```python
from build123d import *

# Parameters (mm, degrees)
CROQUIS1_R              = 8
SALIENTE_EXTRUIR1_DEPTH = 80
CROQUIS2_R              = 11
SALIENTE_EXTRUIR2_DEPTH = 20
CHAFL_N1_SIZE           = 2
CHAFL_N2_SIZE           = 2


with BuildPart() as part:
    # Croquis1 → Saliente-Extruir1 (new body)
    with BuildSketch(Plane(origin=(0, 0, 0), x_dir=(1, 0, 0), z_dir=(0, 1, 0))):
        Circle(CROQUIS1_R)
    extrude(amount=SALIENTE_EXTRUIR1_DEPTH)

    # Croquis2 → Saliente-Extruir2 (add, symmetric)
    with BuildSketch(Plane(origin=(0, 40, 0), x_dir=(1, 0, 0), z_dir=(0, 1, 0))):
        Circle(CROQUIS2_R)
    extrude(amount=SALIENTE_EXTRUIR2_DEPTH, both=True)

    # Chaflán1
    chafl_n1_edges = [part.edges().sort_by_distance(p)[0] for p in [
        (-8, 80, 0),
    ]]
    chamfer(chafl_n1_edges, length=CHAFL_N1_SIZE)

    # Chaflán2
    chafl_n2_edges = [part.edges().sort_by_distance(p)[0] for p in [
        (-8, 0, 0),
    ]]
    chamfer(chafl_n2_edges, length=CHAFL_N2_SIZE)


solid = part.part
```
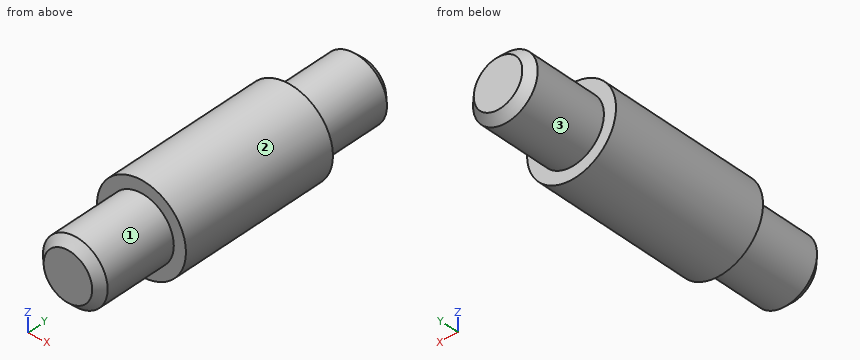
The model under review builds one solid part; all positions refer to its coordinate system, in mm. Face numbers are marked on the shaded views. A direction names the side the tool comes from. Round coordinates to 2 decimals unless told otherwise and drop trailing zeros. Write each loop counter-clockwise with the first axis right and the second up, starting at its lowest first coordinate (ties: lowest second). Pieces come first, ordered by that corner, then holes. Notation, with made-up numbers: M 52.5,-8 L 107.5,-8 A7 cw 107.5,5 Z; hole C 78,79 d8. An arc over 180 degrees is marked long. Use CSV: the item, a comma, the result in double quotes. Start each with the question number.
(1) We need section D-D, the plane y = 23. State the section outline as (x, z) points.
(2) We need section B-B, the plane x = 0. State the section outline as (y, z) points.
(3) We need section C-C, the plane y = 8.5. State the section outline as (x, z) points.
(4) We need section A-A, the plane z = 0. State the section outline as (x, y) points.
(5) Tool access review of the marked faces 1, 2 and 3: name each direction out of +Z, -Z, +X, -X, +Y, -Y from which nothing blocks a thin tool from reaching the whole face with its end or side.
(6) For line 1 along X through (y, z) = (24, -0.25); line 2 along Y through (x, z) = (9, -2.75); line 3 along Z through (x, y) = (-7.25, 41.5), list the stretches that pass through material, from the lowest coordinate up.
(7) Clearance check with flat-ended pins moving along their axes: P1, Ø5, axis at y = 48.5, z = -3.5, coming from the -X side; P2, Ø2, axis at x = 5.5, y = 37.5, coming from the +Z side; P3, Ø1, axis at y = 26, z = -3, coming from the -X side. State where each tip first meets the part, or that it passes through.
Findings:
1,outline,"C 0,0 d22"
2,outline,"M 0,-6 L 2,-8 L 20,-8 L 20,-11 L 60,-11 L 60,-8 L 78,-8 L 80,-6 L 80,6 L 78,8 L 60,8 L 60,11 L 20,11 L 20,8 L 2,8 L 0,6 Z"
3,outline,"C 0,0 d16"
4,outline,"M -11,20 L -8,20 L -8,2 L -6,0 L 6,0 L 8,2 L 8,20 L 11,20 L 11,60 L 8,60 L 8,78 L 6,80 L -6,80 L -8,78 L -8,60 L -11,60 Z"
5,face 1,"-Y"
5,face 2,"+Y, -Y"
5,face 3,"+Y"
6,line 1,"-11 to 11"
6,line 2,"20 to 60"
6,line 3,"-8.27 to 8.27"
7,P1,"x = -10.95"
7,P2,"z = 10.04"
7,P3,"x = -10.71"
